The model under review builds one solid part; all positions refer to its coordinate system, in mm. Face numbers are marked on the shaded views. Round coordinates to 2 decimals unless told otherwise and drop trailing zeros. Loops run counter-clockwise (first coordinate to the right, second up) from the corner with the lowest first, then second, coordinate; pieces in that order, holes last. Notation, with made-up numbers: (56.25, 6.25) - (63.25, 6.25) arc R24 cw to (63.25, 44.25) - close; hole circle Ø6 at (-34, 57). An arc over 180 degrees is marked (long way). Answer as CSV lines item,"result".
from build123d import *

# Parameters (mm, degrees)
SKETCH1_R           = 115
BOSS_EXTRUDE1_DEPTH = 30


with BuildPart() as part:
    # Sketch1 → Boss-Extrude1 (new body)
    with BuildSketch(Plane(origin=(0, 0, 0), x_dir=(1, 0, 0), z_dir=(0, 1, 0))):
        Circle(SKETCH1_R)
        with BuildLine():
            Line((0, 105.05), (0, 97.45))
            ThreePointArc((0, 97.45), (-2.975978112, 97.404548427), (-5.949180178, 97.268236106))
            Line((-5.949180178, 97.268236106), (-5.753824851, 94.074204751))
            ThreePointArc((-5.753824851, 94.074204751), (3.207077785, 94.195420016), (12.138984977, 93.465007055))
            Line((12.138984977, 93.465007055), (12.551130886, 96.638354774))
            ThreePointArc((12.551130886, 96.638354774), (9.59408525, 96.976574636), (6.628090075, 97.224332973))
            Line((6.628090075, 97.224332973), (7.145006284, 104.806733492))
            ThreePointArc((7.145006284, 104.806733492), (43.173122748, 95.768387123), (73.803507095, 74.756570551))
            Line((73.803507095, 74.756570551), (68.429376346, 69.382439802))
            ThreePointArc((68.429376346, 69.382439802), (66.525250753, 71.210206517), (64.572323699, 72.985734991))
            Line((64.572323699, 72.985734991), (62.451939544, 70.589076684))
            ThreePointArc((62.451939544, 70.589076684), (68.8739667, 64.338473801), (74.673298886, 57.506181698))
            Line((74.673298886, 57.506181698), (77.208625745, 59.458646222))
            ThreePointArc((77.208625745, 59.458646222), (75.137185677, 62.055667175), (72.978432671, 64.580576529))
            Line((72.978432671, 64.580576529), (78.705648152, 69.576745031))
            ThreePointArc((78.705648152, 69.576745031), (98.00273537, 37.828115999), (105.041353, 1.347835265))
            Line((105.041353, 1.347835265), (97.44067857, 1.347835265))
            ThreePointArc((97.44067857, 1.347835265), (97.381638194, 3.649526366), (97.268236106, 5.949180178))
            Line((97.268236106, 5.949180178), (94.074204751, 5.753824851))
            ThreePointArc((94.074204751, 5.753824851), (94.206040936, 2.87825487), (94.25, 0))
            ThreePointArc((94.25, 0), (94.053547022, -6.082170053), (93.465007055, -12.138984977))
            Line((93.465007055, -12.138984977), (96.638354774, -12.551130886))
            ThreePointArc((96.638354774, -12.551130886), (97.040462342, -8.92475033), (97.306537269, -5.285858937))
            Line((97.306537269, -5.285858937), (104.889607544, -5.802820805))
            ThreePointArc((104.889607544, -5.802820805), (96.234836599, -42.123137642), (75.423107292, -73.122208571))
            Line((75.423107292, -73.122208571), (70.048400827, -67.747502106))
            ThreePointArc((70.048400827, -67.747502106), (71.534686983, -66.176212178), (72.985734991, -64.572323699))
            Line((72.985734991, -64.572323699), (70.589076684, -62.451939544))
            ThreePointArc((70.589076684, -62.451939544), (64.338473801, -68.8739667), (57.506181698, -74.673298886))
            Line((57.506181698, -74.673298886), (59.458646222, -77.208625745))
            ThreePointArc((59.458646222, -77.208625745), (62.396629618, -74.854279185), (65.241478394, -72.388203438))
            Line((65.241478394, -72.388203438), (70.238137515, -78.115981326))
            ThreePointArc((70.238137515, -78.115981326), (38.241100725, -97.842325787), (1.347835265, -105.041353))
            Line((1.347835265, -105.041353), (1.347835265, -97.44067857))
            ThreePointArc((1.347835265, -97.44067857), (3.649526366, -97.381638194), (5.949180178, -97.268236106))
            Line((5.949180178, -97.268236106), (5.753824851, -94.074204751))
            ThreePointArc((5.753824851, -94.074204751), (-3.207077785, -94.195420016), (-12.138984977, -93.465007055))
            Line((-12.138984977, -93.465007055), (-12.551130886, -96.638354774))
            ThreePointArc((-12.551130886, -96.638354774), (-8.97039747, -97.036253376), (-5.377403168, -97.301521238))
            Line((-5.377403168, -97.301521238), (-5.894359023, -104.884503296))
            ThreePointArc((-5.894359023, -104.884503296), (-42.601180134, -96.024173786), (-73.803507095, -74.756570551))
            Line((-73.803507095, -74.756570551), (-68.429376346, -69.382439802))
            ThreePointArc((-68.429376346, -69.382439802), (-66.525250753, -71.210206517), (-64.572323699, -72.985734991))
            Line((-64.572323699, -72.985734991), (-62.451939544, -70.589076684))
            ThreePointArc((-62.451939544, -70.589076684), (-68.8739667, -64.338473801), (-74.673298886, -57.506181698))
            Line((-74.673298886, -57.506181698), (-77.208625745, -59.458646222))
            ThreePointArc((-77.208625745, -59.458646222), (-75.178448793, -62.005671814), (-73.064286712, -64.48342816))
            Line((-73.064286712, -64.48342816), (-78.791456749, -69.479557018))
            ThreePointArc((-78.791456749, -69.479557018), (-98.2663346, -37.137985733), (-105.05, 0))
            Line((-105.05, 0), (-97.45, 0))
            ThreePointArc((-97.45, 0), (-97.404548427, -2.975978112), (-97.268236106, -5.949180178))
            Line((-97.268236106, -5.949180178), (-94.074204751, -5.753824851))
            ThreePointArc((-94.074204751, -5.753824851), (-94.195420016, 3.207077785), (-93.465007055, 12.138984977))
            Line((-93.465007055, 12.138984977), (-96.638354774, 12.551130886))
            ThreePointArc((-96.638354774, 12.551130886), (-96.972051222, 9.639698217), (-97.218054759, 6.71954826))
            Line((-97.218054759, 6.71954826), (-104.800458391, 7.236464681))
            ThreePointArc((-104.800458391, 7.236464681), (-95.552521618, 43.64880425), (-74.083919205, 74.478691014))
            Line((-74.083919205, 74.478691014), (-68.709887215, 69.104659024))
            ThreePointArc((-68.709887215, 69.104659024), (-70.88404513, 66.872674883), (-72.985734991, 64.572323699))
            Line((-72.985734991, 64.572323699), (-70.589076684, 62.451939544))
            ThreePointArc((-70.589076684, 62.451939544), (-64.338473801, 68.8739667), (-57.506181698, 74.673298886))
            Line((-57.506181698, 74.673298886), (-59.458646222, 77.208625745))
            ThreePointArc((-59.458646222, 77.208625745), (-61.663262597, 75.459555697), (-63.816455081, 73.647556381))
            Line((-63.816455081, 73.647556381), (-68.812532618, 79.374667588))
            ThreePointArc((-68.812532618, 79.374667588), (-36.72324652, 98.422079154), (0, 105.05))
        make_face(mode=Mode.SUBTRACT)
    extrude(amount=BOSS_EXTRUDE1_DEPTH)


solid = part.part
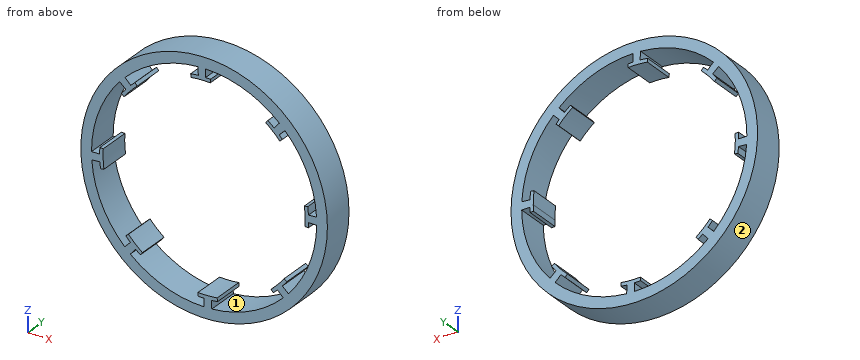
1. Wall thickness on probe 1 along Z at (x, y) = (11.5, 7.75); probe 2 along X at (y, z) = (19.75, -76); probe 3 along X at (y, z) = (5.25, 59): over which ranges is each line inside the solid? List them lowest first.
Numbers:
probe 1,"z = -114.42 to -104.42, -96.77 to -93.55, 104.42 to 114.42"
probe 2,"x = -86.31 to -65.87, -61 to -58.53, 72.52 to 86.31"
probe 3,"x = -98.71 to -86.92, -76.61 to -73.5, 86.92 to 98.71"
2. Clearance check with flat-ended pins moving along their axes: pin 1 (5 mm diameter, centred on y = 13.5, z = -13, fed in from -X); pin 2 (10 mm diameter, centred on x = -87, y = 5, fed in from +Z); pin 3 (8.5 mm diameter, centred on y = 17, z = -103, fed in from -X). State where each tip first meets the part, or that it passes through.
Numbers:
pin 1,"stops at x = -114.52"
pin 2,"stops at z = 80.63"
pin 3,"stops at x = -58.94"
3. Take a section at A-A (z = 39). State the section outline as (x, y) points, plus the area to 3 significant figures.
Numbers:
outline,"(-108.19, 0) - (-97.54, 0) - (-97.54, 30) - (-108.19, 30) - close; (97.54, 0) - (108.19, 0) - (108.19, 30) - (97.54, 30) - close"
area,"639 mm²"
4. Draft analysis for pull direction Z (two halves, no side actions). For the marked faces 1 and 2, state which applies: +Z half, -Z half, draft (parallel to the pull), parting line (faces both ways), or undercut.
Numbers:
face 1,"undercut"
face 2,"parting line"
5. Take a section at B-B (x = -89). State the section outline as (y, z) points.
Numbers:
outline,"(0, -72.83) - (30, -72.83) - (30, -55.81) - (0, -55.81) - close; (0, 55.81) - (30, 55.81) - (30, 72.83) - (0, 72.83) - close"
